Model file for the job. Use its own axes, mm. Face numbers are marked on the shaded views. Round coordinates to 2 decimals unless told otherwise and drop trailing zeros. Order: outer loops, then holes, each group sorted by start corner. A loop starts at its lowest first (then second) coordinate and runs counter-clockwise, first axis right, second up. Notation, with made-up numbers: M 76.25,55.25 L 101.25,55.25 A17 ccw 101.25,59.25 Z; hole C -21,34.25 d6. An arc over 180 degrees is marked long. Return JSON: item names as keys, results as strings. Group by question number.
Item 1: Slice it at C-C on z = 12.7. Write the cut outline in (x, y) (3 decimals), then the cut area to 3 significant figures.
Item 2: Slice it at B-B on y = 42. Write the cut outline in (x, z) (3 decimals).
Item 3: Pull direction Y, two halves, no side cores. Call the marked faces 1, 2 and 3: pulls with the +Y half, pulls with the -Y half, needs draft (parallel to the pull), parting line crosses it, or undercut.
Item 4: Pin check, flat tips, straight feed: pin 1 Ø3.5 at (x, z) = (5.5, 21.5) entering from +Y; pin 2 Ø1 at (y, z) = (21, 9) entering from -X; pin 3 Ø1.1 at (x, z) = (5.5, 19) entering from -Y; pin 4 Ø1.5 at (x, z) = (1, -61.5) entering from -Y. Stop position of each tip, or through.
Item 5: Probe line 1 along Y through (x, z) = (2, -42.5); line 2 along Y through (x, z) = (1.55, -6.35); line 3 along Y through (x, z) = (5, -16). List the from-to ranges inside material, lowest first.
Item 6: Slice it at D-D on y = 0. Write the cut outline in (x, z) (3 decimals).
Item 7: Slice it at A-A on z = 0. Write the cut outline in (x, y) (3 decimals).
Autodesk Inventor part; units mm, degrees
ref_plane "YZ Plane" through (0, 0, 0) normal (1, 0, 0) x (0, 1, 0)
ref_plane "XZ Plane" through (0, 0, 0) normal (0, 1, 0) x (-1, 0, 0)
ref_plane "XY Plane" through (0, 0, 0) normal (0, 0, 1) x (1, 0, 0)
sketch "Sketch1" plane through (0, 0, 0) normal (1, 0, 0) x (0, 1, 0)
  circle A0 centre (0, 0) radius 38.1 construction
  line L0 (27.94, -25.903) -> (27.94, -76.2) construction
  line L1 (27.94, -76.2) -> (-27.94, -76.2) construction
  line L2 (-27.94, -76.2) -> (-27.94, -25.903) construction
  line L3 (-30.1625, -17.4625) -> (30.1625, -17.4625) construction
  line L4 (30.1625, -17.4625) -> (30.1625, 17.4625) construction
  line L5 (30.1625, 17.4625) -> (-30.1625, 17.4625) construction
  line L6 (-30.1625, 17.4625) -> (-30.1625, -17.4625) construction
  line L7 (-30.1625, -17.4625) -> (30.1625, 17.4625) construction
  line L8 (30.1625, -17.4625) -> (-30.1625, 17.4625) construction
  circle A1 centre (30.1625, 17.4625) radius 2.5527 construction
  circle A2 centre (30.1625, -17.4625) radius 2.5527 construction
  circle A3 centre (-30.1625, -17.4625) radius 2.5527 construction
  circle A4 centre (-30.1625, 17.4625) radius 2.5527 construction
  point P0 (0, -76.2)
  dimension "d0" = 76.2
  dimension "d1" = 55.88
  dimension "d2" = 76.2
  dimension "d3" = 60.325
  dimension "d4" = 34.925
  dimension "d5" = 5.1054
  dimension "d6" = 5.1054
  dimension "d7" = 5.1054
  dimension "d8" = 5.1054
sketch "Sketch2" plane through (0, 0, 0) normal (1, 0, 0) x (0, 1, 0)
  line L0 (-30.1625, -17.4625) -> (30.1625, -17.4625) construction
  circle A0 centre (30.1625, -17.4625) radius 2.5527 construction
  circle A1 centre (-30.1625, -17.4625) radius 2.5527 construction
  line L1 (-30.1625, 17.4625) -> (-30.1625, -17.4625) construction
  circle A2 centre (-30.1625, 17.4625) radius 2.5527 construction
  line L2 (30.1625, -17.4625) -> (30.1625, 17.4625) construction
  line L3 (30.1625, -17.4625) -> (-30.1625, 17.4625) construction
  line L4 (30.1625, 17.4625) -> (-30.1625, 17.4625) construction
  line L5 (-30.1625, -17.4625) -> (30.1625, 17.4625) construction
  circle A3 centre (30.1625, 17.4625) radius 2.5527 construction
  circle A4 centre (0, 0) radius 38.1 construction
  line L6 (27.94, -25.903) -> (27.94, -76.2) construction
  line L7 (27.94, -76.2) -> (-27.94, -76.2) construction
  line L8 (-27.94, -76.2) -> (-27.94, -25.903) construction
  circle A5 centre (60.325, 0) radius 12.7 construction
  circle A6 centre (35.56, -51.3927) radius 14.2875
  circle A7 centre (35.56, -51.3927) radius 25.4 construction
  circle A8 centre (60.325, 0) radius 9.525
  circle A9 centre (60.325, 0) radius 22.225 construction
  circle A10 centre (30.1625, 17.4625) radius 8.9027 construction
  circle A11 centre (30.1625, -17.4625) radius 8.9027 construction
  circle A12 centre (-30.1625, -17.4625) radius 8.9027 construction
  circle A13 centre (-30.1625, 17.4625) radius 8.9027 construction
  line L9 (63.2628, 22.03) -> (31.3393, 26.2871)
  line L10 (-39.0652, 17.4625) -> (-39.0652, -17.4625)
  arc A14 (80.6974, -8.8835) -> (63.2628, 22.03) centre (60.325, 0) ccw
  arc A15 (31.3393, 26.2871) -> (31.8447, 26.2048) centre (30.1625, 17.4625) ccw
  arc A16 (-31.8447, 26.2048) -> (-39.0652, 17.4625) centre (-30.1625, 17.4625) ccw
  arc A17 (-39.0652, -17.4625) -> (-33.6268, -25.6635) centre (-30.1625, -17.4625) ccw
  circle A18 centre (35.56, -51.3927) radius 25.4 construction
  circle A19 centre (17.331, -33.7048) radius 4.7625 construction
  circle A20 centre (32.8295, -73.6177) radius 4.8895 construction
  circle A21 centre (59.9927, -44.45) radius 4.7625 construction
  circle A22 centre (0, 0) radius 25.4
  circle A23 centre (0, 0) radius 31.75 construction
  line L11 (31.8447, 26.2048) -> (5.9993, 31.178)
  line L12 (-5.9993, 31.178) -> (-31.8447, 26.2048)
  arc A24 (5.9993, 31.178) -> (-5.9993, 31.178) centre (0, 0) ccw
  circle A25 centre (35.56, -51.3927) radius 29.9974 construction
  circle A26 centre (35.56, -51.3927) radius 20.6375 construction
  circle A27 centre (35.56, -51.3927) radius 7.62 construction
  line L13 (80.6974, -8.8835) -> (64.3582, -46.3536)
  line L14 (63.8721, -47.2125) -> (52.3707, -63.3638)
  arc A28 (63.8721, -47.2125) -> (64.3582, -46.3536) centre (59.9927, -44.45) ccw
  arc A29 (19.8728, -64.8023) -> (-33.6268, -25.6635) centre (-89.741, -158.5012) ccw
  arc A30 (19.8728, -64.8023) -> (52.3707, -63.3638) centre (35.56, -51.3927) ccw
  point P0 (0, -76.2)
  point P1 (71.3235, -6.35)
  point P2 (71.3235, 6.35)
  point P3 (60.325, 12.7)
  point P4 (49.3265, 6.35)
  point P5 (49.3265, -6.35)
  point P6 (60.325, -12.7)
  point P7 (29.3562, -76.0235)
  point P8 (31.5932, 26.2532)
  dimension "d9" = 25.4
  dimension "d76" = 50.8
  dimension "d14" = 360
  dimension "d16" = 28.575
  dimension "d17" = 57.0484
  dimension "d19" = 50.8
  dimension "d20" = 19.05
  dimension "d23" = 6.35
  dimension "d43" = 360
  dimension "d45" = 9.525
  dimension "d46" = 9.779
  dimension "d47" = 9.525
  dimension "d56" = 50.8
  dimension "d57" = 6.35
  dimension "d58" = 44.45
  dimension "d60" = 76.2
  dimension "d65" = 59.9948
  dimension "d66" = 6.35
  dimension "d75" = 15.24
  dimension "d77" = 22.225
  dimension "d78" = 44.45
extrude "Extrusion1" add sketch "Sketch2" along normal blind 6.35 contours L11 A15 L9 | A14 L13 A28 L14 A30 A29 A17 L10 A16 L12 A24 L11 L9
hole "Motor Mount Holes" at (0, -30.1625, -17.4625) at (0, 30.1625, -17.4625) at (0, -30.1625, 17.4625) at (0, 30.1625, 17.4625) at (0, 0, -76.2) at (0, 71.3235, -6.35) at (0, 71.3235, 6.35) at (0, 60.325, 12.7) at (0, 49.3265, 6.35) at (0, 49.3265, -6.35) at (0, 60.325, -12.7) direction (1, 0, 0) diameter 4.9784 end through all
hole "Hole3" at (0, 59.9927, -44.45) direction (1, 0, 0) diameter 4.9784 end through all
sketch "Sketch3" plane through (6.35, 0, 0) normal (1, 0, 0) x (0, 0, -1)
  circle A0 centre (0, 60.325) radius 9.525
  circle A1 centre (0, 60.325) radius 20.32
  point P0 (0, 0)
  dimension "d61" = 40.64
extrude "Extrusion2" cut sketch "Sketch3" against normal blind 3.175
sketch "Sketch4" plane through (6.35, 0, 0) normal (1, 0, 0) x (0, 0, -1)
  circle A0 centre (0, 60.325) radius 20.32
  circle A1 centre (44.45, 59.9927) radius 2.4892
  circle A2 centre (-17.4625, 30.1625) radius 2.4892
  circle A3 centre (17.4625, 30.1625) radius 2.4892
  circle A4 centre (17.4625, -30.1625) radius 2.4892
  circle A5 centre (-17.4625, -30.1625) radius 2.4892
  circle A6 centre (51.3927, 35.56) radius 14.2875
  circle A7 centre (0, 0) radius 25.4
  line L0 (17.4625, -39.0652) -> (-17.4625, -39.0652)
  arc A8 (-26.2048, -31.8447) -> (-17.4625, -39.0652) centre (-17.4625, -30.1625) ccw
  line L1 (-26.2048, -31.8447) -> (-31.178, -5.9993)
  arc A9 (-31.178, 5.9993) -> (-31.178, -5.9993) centre (0, 0) ccw
  line L2 (-31.178, 5.9993) -> (-26.2532, 31.5932)
  line L3 (-26.2532, 31.5932) -> (-22.03, 63.2628)
  arc A10 (8.8835, 80.6974) -> (-22.03, 63.2628) centre (0, 60.325) ccw
  line L4 (-20.0805, 69.85) -> (-17.9493, 69.85)
  circle A11 centre (0, 60.325) radius 20.32
  line L5 (-22.03, 63.2628) -> (-26.2532, 31.5932)
  line L6 (-23.6919, 50.8) -> (-17.9493, 50.8)
  arc A12 (8.8835, 80.6974) -> (-22.03, 63.2628) centre (0, 60.325) ccw
  line L7 (8.8835, 80.6974) -> (46.3536, 64.3582)
  arc A13 (47.2125, 63.8721) -> (46.3536, 64.3582) centre (44.45, 59.9927) ccw
  line L8 (47.2125, 63.8721) -> (63.3638, 52.3707)
  arc A14 (64.8023, 19.8728) -> (25.6635, -33.6268) centre (158.5012, -89.741) ccw
  arc A15 (17.4625, -39.0652) -> (25.6635, -33.6268) centre (17.4625, -30.1625) ccw
  arc A16 (64.8023, 19.8728) -> (63.3638, 52.3707) centre (51.3927, 35.56) ccw
  point P0 (5.7277, 81.7993)
  point P1 (-20.8206, 50.8)
  point P2 (-19.0149, 69.85)
  dimension "d68" = 19.05
  dimension "d69" = 9.525
extrude "Extrusion3" cut sketch "Sketch4" against normal blind 3.175 contours A0 L6 L3 A10 L4
sketch "Sketch5" plane through (0, 0, 0) normal (-1, 0, 0) x (0, 0, 1)
  circle A0 centre (0, 0) radius 22.225
  circle A1 centre (0, 0) radius 25.4
  dimension "d72" = 44.45
extrude "Extrusion4" add sketch "Sketch5" against normal blind 2.54
properties part number "AR-002" material "Aluminum 6061"
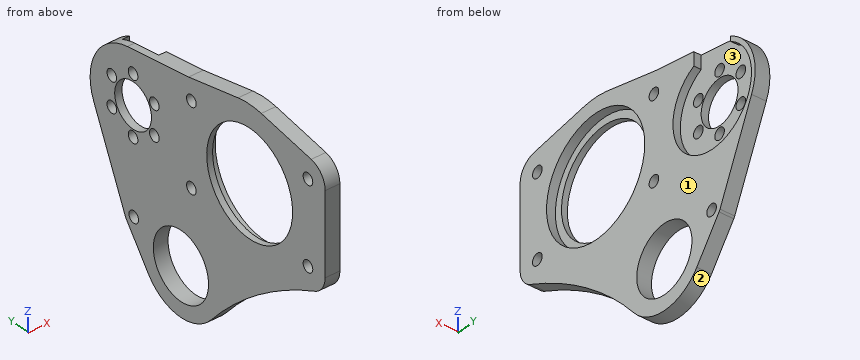
Output values:
{
 "1": {"outline": "M 0,-39.065 L 6.35,-39.065 L 6.35,-21.997 L 2.54,-21.997 L 2.54,-18.239 L 0,-18.239 Z; M 0,18.239 L 2.54,18.239 L 2.54,21.997 L 6.35,21.997 L 6.35,44.463 L 3.175,44.463 L 3.175,57.836 L 0,57.836 Z; M 0,62.814 L 3.175,62.814 L 3.175,76.187 L 6.35,76.187 L 6.35,78.564 L 0,78.564 Z", "area": "370 mm²"},
 "2": {"outline": "M 0,-71 L 6.35,-71 L 6.35,-64.146 L 0,-64.146 Z; M 0,-38.639 L 6.35,-38.639 L 6.35,-8.78 L 3.175,-8.78 L 3.175,8.78 L 6.35,8.78 L 6.35,24.865 L 0,24.865 Z"},
 "3": {"face 1": "needs draft", "face 2": "parting line crosses it", "face 3": "undercut"},
 "4": {"pin 1": "y = 70.52", "pin 2": "x = 0", "pin 3": "y = -39.01", "pin 4": "y = 16.27"},
 "5": {"line 1": "-4.08 to 24.38, 46.74 to 58.45, 61.54 to 66.04", "line 2": "-39.07 to -21.3, 21.3 to 46.84, 51.82 to 53.23, 67.42 to 68.83, 73.81 to 81.62", "line 3": "-39.07 to -32.18, -28.15 to -19.73, 19.73 to 28.15, 32.18 to 47.8, 72.85 to 77.59"},
 "6": {"outline": "M 0,-45.624 L 6.35,-45.624 L 6.35,-25.4 L 2.54,-25.4 L 2.54,-22.225 L 0,-22.225 Z; M 0,22.225 L 2.54,22.225 L 2.54,25.4 L 6.35,25.4 L 6.35,31.75 L 0,31.75 Z"},
 "7": {"outline": "M 0,-39.065 L 6.35,-39.065 L 6.35,-25.4 L 2.54,-25.4 L 2.54,-22.225 L 0,-22.225 Z; M 0,22.225 L 2.54,22.225 L 2.54,25.4 L 6.35,25.4 L 6.35,40.005 L 3.175,40.005 L 3.175,50.8 L 0,50.8 Z; M 0,69.85 L 3.175,69.85 L 3.175,80.645 L 6.35,80.645 L 6.35,82.55 L 0,82.55 Z"}
}
